The model under review builds one solid part; all positions refer to its coordinate system, in mm. Face numbers are marked on the shaded views. A direction names the side the tool comes from. Coordinates: 2 decimals unless noted, no trailing zeros. Loops run counter-clockwise (first coordinate to the right, second up) from the corner with the lowest first, then second, coordinate; pieces in that order, holes last. Notation, with made-up numbers: (-32.5, 42) -> (-1.5, 42) arc R21 cw to (-1.5, 51) -> close; hole circle Ø9 at (-3.75, 41.5). An arc over 180 degrees is marked (long way). One line per question, with ' | ' between items. Start each with the question number.
from build123d import *

# Parameters (mm, degrees)
F0_R     = 5
F1_DEPTH = 5
F2_W     = 260
F2_H     = 5
F3_DEPTH = 27
F4_R     = 16
F6_DEPTH = 5
F7_R     = 2


with BuildPart() as f1:
    # F0 (on Top) → F1 (new body)
    with BuildSketch(Plane.XY):
        with BuildLine():
            Line((130, -28), (130, 0))
            Line((130, 0), (-130, 0))
            Line((-130, 0), (-130, -28))
            ThreePointArc((-130, -28), (-125.313708499, -39.313708499), (-114, -44))
            Line((-114, -44), (114, -44))
            ThreePointArc((114, -44), (125.313708499, -39.313708499), (130, -28))
        make_face()
        with Locations((-114, -28)):
            Circle(F0_R, mode=Mode.SUBTRACT)
        with Locations((-88, -28)):
            Circle(F0_R, mode=Mode.SUBTRACT)
        with BuildLine():
            Line((12, -23), (114, -23))
            ThreePointArc((114, -23), (119, -28), (114, -33))
            Line((114, -33), (12, -33))
            ThreePointArc((12, -33), (7, -28), (12, -23))
        make_face(mode=Mode.SUBTRACT)
    extrude(amount=-F1_DEPTH)

    # F2 (on face) → F3 (join)
    with BuildSketch(Plane(origin=(0, 0, -5), x_dir=(1, 0, 0), z_dir=(0, 0, -1))):
        with Locations((0, 2.5)):
            Rectangle(F2_W, F2_H)
    extrude(amount=F3_DEPTH)

    # F4
    f4_edges = [f1.edges().sort_by_distance(p)[0] for p in [
        (130, -2.5, -32),
        (-130, -2.5, -32),
    ]]
    fillet(f4_edges, radius=F4_R)

    # F5 (on face) → F6 (cut)
    with BuildSketch(Plane(origin=(0, 0, 0), x_dir=(-1, 0, 0), z_dir=(0, 1, 0))):
        with BuildLine():
            ThreePointArc((48, -24), (54, -18), (48, -12))
            Line((48, -12), (-112, -12))
            ThreePointArc((-112, -12), (-118, -18), (-112, -24))
            Line((-112, -24), (48, -24))
        make_face()
    extrude(amount=-F6_DEPTH, mode=Mode.SUBTRACT)

    # F7
    f7_edges = [f1.edges().sort_by_distance(p)[0] for p in [
        (0, 0, -32),
        (-125.313708, -5, -27.313708),
        (0, -5, -5),
        (130, -5, -10.5),
        (130, -16.5, -5),
        (130, 0, -8),
        (125.313708, -5, -27.313708),
        (0, -5, -32),
        (-130, -5, -10.5),
        (125.313708, 0, -27.313708),
        (125.313708, -39.313708, -5),
        (0, -44, -5),
        (-125.313708, -39.313708, -5),
        (-130, -16.5, -5),
        (-130, 0, -8),
        (-125.313708, 0, -27.313708),
    ]]
    fillet(f7_edges, radius=F7_R)


solid = f1.part
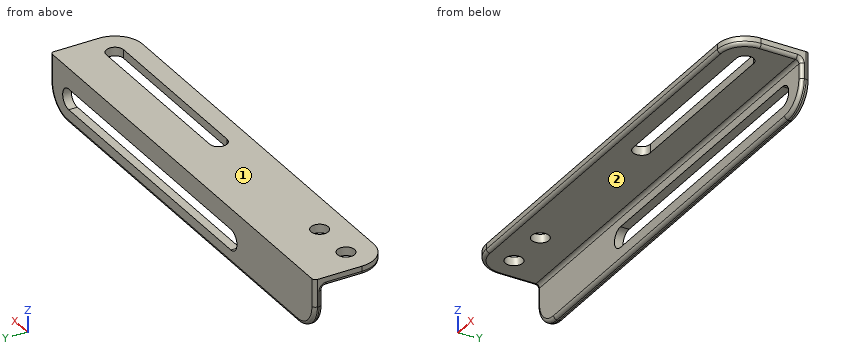
1) Machinability: for the marked faces 1 and 2, which of the approach directions +Z, -Z, +X, -X, +Y, -Y give a long, thin tool a straight path to every point of the face, cutting with its end or side? Answer none if there is none.
2) Consider section B-B, the plane y = -20. Write out the cut boundary in (x, z).
3) Insertion check: pin 1 Ø1 at (x, y) = (86.5, -35) entering from -Z; pin 2 Ø1 at (x, z) = (-26, -9.5) entering from -Y. Each pin has a flat end and moves straight along its axis. Give the tip position at first contact, or say it passes through.
4) Consider section A-A, the plane x = 87. Write out the cut boundary in (y, z).
5) Wall thickness on L1, parallel to Y at x = -88, z = -2.7; L2, parallel to Z at x = -41, y = -3; L3, parallel to Y at x = -86, z = -29: over which ranges is each line inside the solid? List them lowest first.
Filled sheet:
1) face 1: +Z, +X, -X, +Y, -Y | face 2: -Z, +X, -X, -Y
2) outline: (-130, -3) arc R2 ccw to (-128, -5) -> (128, -5) arc R2 ccw to (130, -3) -> (130, 0) -> (-130, 0) -> close
3) pin 1: z = -5 | pin 2: y = -5
4) outline: (-44, -3) arc R2 ccw to (-42, -5) -> (-33, -5) -> (-33, 0) -> (-44, 0) -> close; (-23, -5) -> (-7, -5) arc R2 cw to (-5, -7) -> (-5, -12) -> (0, -12) -> (0, 0) -> (-23, 0) -> close; (-5, -30) arc R2 ccw to (-3, -32) -> (-2, -32) arc R2 ccw to (0, -30) -> (0, -24) -> (-5, -24) -> close
5) L1: -44 to -33, -23 to 0 | L2: -32 to -24, -12 to 0 | L3: -5 to 0
